Build history of the part. All positions in model axes, mm. A direction names the side the tool comes from. Give positions to 0.01 mm unless a question says otherwise; leave off trailing zeros. Loops run counter-clockwise (first coordinate to the right, second up) from the corner with the lowest first, then second, coordinate; pieces in that order, holes last. Notation, with made-up numbers: (35.25, 84) - (83.25, 84) arc R24 ccw to (83.25, 95) - close; hole circle Ø6 at (32, 13). An arc over 180 degrees is marked (long way). Return JSON: item names as keys, results as strings. Group by question number.
1) Slice it at D-D (x = -1.5). List the corners of the cut face in (y, z).
2) Drop flat-ended pins along their axis: pin 1 (5.5 mm diameter, centred on x = -3, z = -10, fed in from -Y); pin 2 (5 mm diameter, centred on x = -1, y = 1, fed in from -Z). Give the stop position or say it passes through.
3) Slice it at C-C (y = -7). List the corners of the cut face in (x, z).
4) 3-axis set-ups, long thin cutter, end or side, ignore diameter. For faces 5 (the face through (-10, 9, 0)), 6 (the face through (0, -1, 0)): which of +Z, -Z, +X, -X, +Y, -Y reach the whole face in a straight line?
5) Mould opens along X. For faces 1 (the face through (0, 22, -6)), 2 (the face through (6.386, -6.727, 2.958)), 3 (the face through (-6.19, 2.935, 2.958)), 4 (the face through (7.9, 14.6, -16)) say: released by +X, released by -X, zero draft, split by the parting line, or undercut.
6) Slice it at B-B (x = -5). List the corners of the cut face in (y, z).
7) Drill centre lines: probe 1 along Y at (x, z) = (-5, 1.45); probe 2 along Y at (x, z) = (5.5, 3.75); probe 3 along Z at (x, y) = (-1, -6.5). Where is each one in solid material? Low to high. Write a range as from..to.
8) Slice it at A-A (y = 20.5). List the corners of the cut face in (x, z).
```python
from build123d import *

# Parameters (mm, degrees)
SKETCH_1_W          = 20
SKETCH_1_H          = 20
SKETCH_1_R          = 1.5
EXTRUDE_1_DEPTH     = 6
SKETCH_2_W          = 20
SKETCH_2_H          = 3
EXTRUDE_2_DEPTH     = 18
SKETCH_3_W          = 20
SKETCH_3_H          = 24
EXTRUDE_3_DEPTH     = 12
CUT_EXTRUDE_1_DEPTH = 39.052595181


with BuildPart() as part:
    # Эскиз1 → Бобышка-Вытянуть1 (new body)
    with BuildSketch(Plane.XY):
        Rectangle(SKETCH_1_W, SKETCH_1_H)
        with Locations((-5, -6.152042824)):
            Circle(SKETCH_1_R, mode=Mode.SUBTRACT)
        with Locations((-5, 3.847957176)):
            Circle(SKETCH_1_R, mode=Mode.SUBTRACT)
        with Locations((5, 3.847957176)):
            Circle(SKETCH_1_R, mode=Mode.SUBTRACT)
        with Locations((5, -6.152042824)):
            Circle(SKETCH_1_R, mode=Mode.SUBTRACT)
    extrude(amount=EXTRUDE_1_DEPTH)

    # Эскиз2 → Бобышка-Вытянуть2 (add)
    with BuildSketch(Plane(origin=(0, 0, 0), x_dir=(-1, 0, 0), z_dir=(0, 0, -1))):
        with Locations((0, 8.5)):
            Rectangle(SKETCH_2_W, SKETCH_2_H)
    extrude(amount=EXTRUDE_2_DEPTH)

    # Эскиз3 → Бобышка-Вытянуть3 (add)
    with BuildSketch(Plane(origin=(0, 10, 0), x_dir=(1, 0, 0), z_dir=(0, 1, 0))):
        with Locations((0, 6)):
            Rectangle(SKETCH_3_W, SKETCH_3_H)
    extrude(amount=EXTRUDE_3_DEPTH)

    # Эскиз4 → Вырез-Вытянуть1 (cut, through all)
    with BuildSketch(Plane(origin=(0, 22, 0), x_dir=(1, 0, 0), z_dir=(0, 1, 0))):
        with BuildLine():
            Line((-10, 18), (-10, 11))
            ThreePointArc((-10, 11), (-7.949747468, 15.949747468), (-3, 18))
            Line((-3, 18), (-10, 18))
        make_face()
        with BuildLine():
            ThreePointArc((0, 12.591020059), (-2, 10.591020059), (0, 8.591020059))
            Line((0, 8.591020059), (0, 12.591020059))
        make_face()
        with BuildLine():
            Line((0, 12.591020059), (0, 8.591020059))
            ThreePointArc((0, 8.591020059), (1.414213562, 9.176806496), (2, 10.591020059))
            ThreePointArc((2, 10.591020059), (1.414213562, 12.005233621), (0, 12.591020059))
        make_face()
        with BuildLine():
            ThreePointArc((3, 18), (7.949747468, 15.949747468), (10, 11))
            Line((10, 11), (10, 18))
            Line((10, 18), (3, 18))
        make_face()
    extrude(amount=-CUT_EXTRUDE_1_DEPTH, mode=Mode.SUBTRACT)


solid = part.part
```
Results:
{
 "1": {"outline": "(-10, 0) - (7, 0) - (7, -9.27) - (22, -9.27) - (22, 6) - (-10, 6) - close; (7, -18) - (22, -18) - (22, -11.91) - (7, -11.91) - close"},
 "2": {"pin 1": "y = 7", "pin 2": "z = 0"},
 "3": {"outline": "(-10, 0) - (-6.24, 0) - (-6.24, 6) - (-10, 6) - close; (-3.76, 0) - (3.76, 0) - (3.76, 6) - (-3.76, 6) - close; (6.24, 0) - (10, 0) - (10, 6) - (6.24, 6) - close"},
 "4": {"face 5": "+Z, -Z, -X, +Y, -Y", "face 6": "-Z, +X, -X, -Y"},
 "5": {"face 1": "zero draft", "face 2": "undercut", "face 3": "undercut", "face 4": "released by +X"},
 "6": {"outline": "(-10, 0) - (-7.65, 0) - (-7.65, 6) - (-10, 6) - close; (-4.65, 0) - (2.35, 0) - (2.35, 6) - (-4.65, 6) - close; (5.35, 0) - (7, 0) - (7, -17.71) - (22, -17.71) - (22, 6) - (5.35, 6) - close"},
 "7": {"probe 1": "-10..-7.65, -4.65..2.35, 5.35..22", "probe 2": "-10..-7.57, -4.74..2.43, 5.26..22", "probe 3": "0..6"},
 "8": {"outline": "(-10, -11) arc R7 ccw to (-3, -18) - (3, -18) arc R7 ccw to (10, -11) - (10, 6) - (-10, 6) - close; hole circle Ø4 at (0, -10.59)"}
}
